Model file for the job. Use its own axes, mm. Face numbers are marked on the shaded views. Give positions to 0.01 mm unless a question says otherwise; leave off trailing zeros. Write each loop counter-clockwise with the first axis right and the second up, starting at its lowest first coordinate (ties: lowest second). Pieces come first, ordered by that corner, then holes. Notation, with made-up numbers: (-10, 40.5) - (28, 40.5) arc R23 cw to (28, 54.5) - close; hole circle Ø2 at (46.5, 45). An arc over 180 degrees is marked (long way). Use CSV: the item, a comma, the result in double quotes.
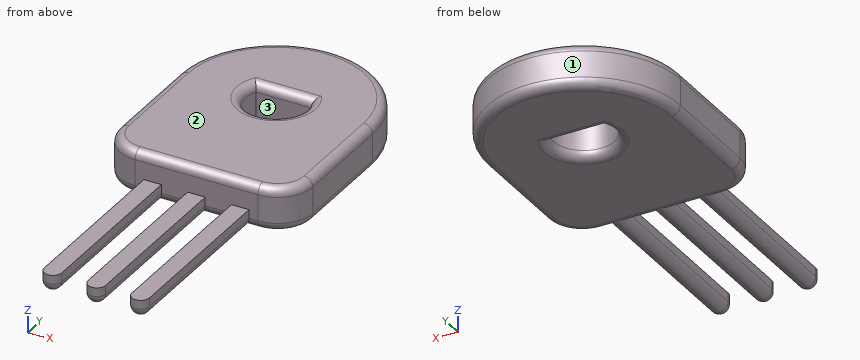
from build123d import *

# Parameters (mm, degrees)
BOSS_EXTRUDE1_DEPTH = 2.5
BOSS_EXTRUDE2_DEPTH = 1
FILLET1_R           = 2
FILLET2_R           = 0.5


with BuildPart() as part:
    # Sketch1 → Boss-Extrude1 (new body)
    with BuildSketch(Plane.XY):
        with BuildLine():
            Line((5.5, 0), (5.5, -8))
            Line((5.5, -8), (-5.5, -8))
            Line((-5.5, -8), (-5.5, 0))
            ThreePointArc((-5.5, 0), (0, 5.5), (5.5, 0))
        make_face()
        with BuildLine():
            ThreePointArc((-1.58113883, 0.75), (0, -1.75), (1.58113883, 0.75))
            Line((1.58113883, 0.75), (-1.58113883, 0.75))
        make_face(mode=Mode.SUBTRACT)
    extrude(amount=BOSS_EXTRUDE1_DEPTH)

    # Sketch1<3> → Boss-Extrude2 (add)
    with BuildSketch(Plane.XY):
        with BuildLine():
            Line((-2, -8), (-3, -8))
            Line((-3, -8), (-3, -18))
            ThreePointArc((-3, -18), (-2.5, -18.5), (-2, -18))
            Line((-2, -18), (-2, -8))
        make_face()
        with BuildLine():
            Line((0.5, -8), (-0.5, -8))
            Line((-0.5, -8), (-0.5, -18))
            ThreePointArc((-0.5, -18), (0, -18.5), (0.5, -18))
            Line((0.5, -18), (0.5, -8))
        make_face()
        with BuildLine():
            Line((3, -18), (3, -8))
            Line((3, -8), (2, -8))
            Line((2, -8), (2, -18))
            ThreePointArc((2, -18), (2.5, -18.5), (3, -18))
        make_face()
    extrude(amount=BOSS_EXTRUDE2_DEPTH)

    # Fillet1
    fillet1_edges = [part.edges().sort_by_distance(p)[0] for p in [
        (5.5, -8, 1.25),
        (-5.5, -8, 1.25),
    ]]
    fillet(fillet1_edges, radius=FILLET1_R)

    # Fillet2
    fillet2_edges = [part.edges().sort_by_distance(p)[0] for p in [
        (0, 0.75, 2.5),
        (0, -1.75, 0),
        (5.5, -3, 2.5),
        (0, 5.5, 2.5),
        (-3.25, -8, 0),
        (-3, -13, 0),
        (-5.5, -3, 2.5),
        (-2.5, -18.5, 0),
        (-2, -13, 0),
        (-1.25, -8, 0),
        (-0.5, -13, 0),
        (0, -18.5, 0),
        (0.5, -13, 0),
        (1.25, -8, 0),
        (2, -13, 0),
        (2.5, -18.5, 0),
        (3, -13, 0),
        (3.25, -8, 0),
        (-4.914213562, -7.414213562, 0),
        (4.914213562, -7.414213562, 0),
        (0, -8, 2.5),
        (0, -1.75, 2.5),
        (-4.914213562, -7.414213562, 2.5),
        (4.914213562, -7.414213562, 2.5),
        (-5.5, -3, 0),
        (0, 5.5, 0),
        (5.5, -3, 0),
        (0, 0.75, 0),
    ]]
    fillet(fillet2_edges, radius=FILLET2_R - 0.0001)  # a hair under: the kernel refuses the full size


solid = part.part
(1) Saw through at A-A, the plane z = 1.7. List the corners of the cut face in (x, y), then the cut area to 3 significant figures.
Checked values:
outline,"(-5.5, -6) arc R2 ccw to (-3.5, -8) - (3.5, -8) arc R2 ccw to (5.5, -6) - (5.5, 0) arc R5.5 ccw to (-5.5, 0) - close; hole (-1.58, 0.75) arc R1.75 ccw (long way) to (1.58, 0.75) - close"
area,"126 mm^2"
(2) Flat gauge pins, fed straight in: P1, Ø3, axis at x = 0, y = 0, coming from the +Z side; P2, Ø1, axis at x = 4, z = 2, coming from the -Y side; P3, Ø0.8, axis at x = 2.5, y = -12.5, coming from the +Z side; P4, Ø1.5, axis at y = -11.5, z = 2, coming from the +X side. Where does each tip first touch, or does it go through?
Checked values:
P1,"stops at z = 2.5"
P2,"stops at y = -8"
P3,"stops at z = 1"
P4,"passes through"
(3) Saw through at B-B, the plane y = -13. Count the separate pieces of the cut face and the enclosed holes in it, then the cut area to 3 significant figures.
Checked values:
separate pieces,"3"
enclosed holes,"0"
area,"2.68 mm^2"
(4) Wall check: probe 1 along X at (y, z) = (0, 1.65); probe 2 along X at (y, z) = (-10.25, 0.25); probe 3 along Z at (x, y) = (-2.5, -13). Give the ranges that are in metal, low to high. Write a range as [from, to].
Checked values:
probe 1,"x = [-5.5, -1.75], [1.75, 5.5]"
probe 2,"x = [-2.93, -2.07], [-0.43, 0.43], [2.07, 2.93]"
probe 3,"z = [0, 1]"
(5) Pull direction Y, two halves, no side cores. Call the marked faces 1, 2 and 3: released by +Y, released by -Y, zero draft, split by the parting line, or undercut.
Checked values:
face 1,"released by +Y"
face 2,"zero draft"
face 3,"undercut"
